Design review of the part built by this model. Coordinates are the model's own, in mm. A direction names the side the tool comes from. Coordinates: 2 decimals unless noted, no trailing zeros. Write each loop counter-clockwise with the first axis right and the second up, starting at its lowest first coordinate (ties: lowest second). Pieces come first, ordered by that corner, then holes. Notation, with made-up numbers: (-12.5, 85.25) -> (12.5, 85.25) arc R19 ccw to (12.5, 114.25) -> close; hole circle Ø11 at (72, 85.25). An arc over 180 degrees is marked (long way). One line per question, with ' | ' between items. Start each with the question number.
Q1. Draft analysis for pull direction X (two halves, no side actions). For faces 1 (the flat face through (4.762, 10, 2)), 2 (the flat face through (-9.525, -2, 2)), 3 (the flat face through (-4.762, 10, 2)), 4 (the flat face through (9.525, -2, 2)), state which applies: pulls with the +X half, pulls with the -X half, needs draft (parallel to the pull), parting line crosses it, or undercut.
Q2. Add section A-A on x = 0. State the section outline as (y, z) points (1 decimal).
Q3. For P1, Ø1, axis at y = -3, z = 1.5, coming from the +X side; P2, Ø1, axis at x = 8.5, z = 1, coming from the +Y side; P3, Ø1.6, axis at x = -8.5, z = 1.5, coming from the -Y side; P4, Ø10, axis at x = -8.5, y = 2.5, coming from the -Z side, all flat-tipped, find the tip position at first contact; note any pin that passes through.
Q4. Add section C-C on z = 2. Give the number of separate pieces and of enclosed holes in the cut face, and give its area (3 significant figures).
Q5. For faces 5 (the flat face through (-7, 7.938, 2)), 6 (the flat face through (7, 7.938, 2)), 7 (the flat face through (-6.35, -2, 2)), 8 (the flat face through (0, -3, 3.175)), list the 3-axis set-ups (+Z, -Z, +X, -X, +Y, -Y) from which the entire face can be reached by the end or side of a thin tool; tool diameter is ignored.
Q6. Add section D-D on y = 8.25. State the section outline as (x, z) points (1 decimal), and give its area (3 significant figures).
Q7. Wall thickness on probe 1 along X at (y, z) = (-13.5, 2.25); probe 2 along Y at (x, z) = (7, 2); probe 3 along X at (y, z) = (8, 3): over which ranges is each line inside the solid? List them lowest first.
Q8. Add section B-B on y = 0.5. State the section outline as (x, z) points (3 decimals).
from build123d import *

# Parameters (mm, degrees)
SKETCH1_W           = 9.525
SKETCH1_H           = 3.175
SKETCH1_R           = 2.38125
BOSS_EXTRUDE1_DEPTH = 3.175
CAVITY1_START       = -9.525
CAVITY1_OUTLINE_W   = 6.35
CAVITY1_OUTLINE_H   = 3.175
CAVITY1_DEPTH       = 3.175
CAVITY1_START_2     = 6.35
CAVITY1_2_OUTLINE_W = 6.35
CAVITY1_2_OUTLINE_H = 3.175
CAVITY1_2_DEPTH     = 3.175


# Read off the part's stored shape, not the designer's step: Cavity1
with BuildPart() as part:
    # Sketch1 → Boss-Extrude1 (new body)
    # profile 1 of 10: a face of its own
    with BuildSketch(Plane.XY):
        with BuildLine():
            ThreePointArc((-9.525, 7.9375), (-11.876811414, 4.274474566), (-12.7, 0))
            Line((-12.7, 0), (-9.525, 0))
            Line((-9.525, 0), (-9.525, 7.9375))
        make_face()
    # profile 2 of 10: a face of its own
    with BuildSketch(Plane.XY):
        with BuildLine():
            Line((-9.525, 0), (-12.7, 0))
            ThreePointArc((-12.7, 0), (-11.876811414, -4.274474566), (-9.525, -7.9375))
            Line((-9.525, -7.9375), (-9.525, 0))
        make_face()
    # profile 3 of 10: a face of its own
    with BuildSketch(Plane.XY):
        Polygon((-9.525, 7.9375), (-9.525, 0), (0, 0), (9.525, 0), (9.525, 7.9375), (4.7625, 7.9375), (-4.7625, 7.9375), align=None)
    # profile 4 of 10: a face of its own
    with BuildSketch(Plane.XY):
        Polygon((0, 0), (-9.525, 0), (-9.525, -7.9375), (0, -7.9375), (9.525, -7.9375), (9.525, 0), align=None)
    # profile 5 of 10: a face of its own
    with BuildSketch(Plane.XY):
        with BuildLine():
            Line((0, -7.9375), (-9.525, -7.9375))
            add(Edge.make_bspline(
                [(-9.525, -7.9375), (-8.354743729, -9.166269084), (-6.479229503, -10.75772626), (-5.396989703, -14.77189499), (-3.721125314, -16.086113374), (-2.300921541, -16.869792119)],
                knots=[0, 0, 0, 0, 0.40377748, 0.653864755, 1, 1, 1, 1], degree=3))
            ThreePointArc((-2.300921541, -16.869792119), (-4.611943257, -11.511982474), (0, -7.9375))
        make_face()
    # profile 6 of 10: a face of its own
    with BuildSketch(Plane.XY):
        with Locations((0, 9.525)):
            Rectangle(SKETCH1_W, SKETCH1_H)
    # profile 7 of 10: a face of its own
    with BuildSketch(Plane.XY):
        with BuildLine():
            Line((9.525, -7.9375), (0, -7.9375))
            ThreePointArc((0, -7.9375), (3.367596045, -9.332403955), (4.7625, -12.7))
            ThreePointArc((4.7625, -12.7), (4.1011916, -15.121081103), (2.300921541, -16.869792119))
            add(Edge.make_bspline(
                [(9.525, -7.9375), (8.354743729, -9.166269084), (6.479229503, -10.75772626), (5.396989703, -14.77189499), (3.721125314, -16.086113374), (2.300921541, -16.869792119)],
                knots=[0, 0, 0, 0, 0.40377748, 0.653864755, 1, 1, 1, 1], degree=3))
        make_face()
    # profile 8 of 10: a face of its own
    with BuildSketch(Plane.XY):
        with BuildLine():
            ThreePointArc((4.7625, -12.7), (3.367596045, -9.332403955), (0, -7.9375))
            ThreePointArc((0, -7.9375), (-4.611943257, -11.511982474), (-2.300921541, -16.869792119))
            ThreePointArc((-2.300921541, -16.869792119), (0, -17.4625), (2.300921541, -16.869792119))
            ThreePointArc((2.300921541, -16.869792119), (4.1011916, -15.121081103), (4.7625, -12.7))
        make_face()
        with Locations((0, -12.7)):
            Circle(SKETCH1_R, mode=Mode.SUBTRACT)
    # profile 9 of 10: a face of its own
    with BuildSketch(Plane.XY):
        with BuildLine():
            Line((9.525, 7.9375), (9.525, 0))
            Line((9.525, 0), (12.7, 0))
            ThreePointArc((12.7, 0), (11.876811414, 4.274474566), (9.525, 7.9375))
        make_face()
    # profile 10 of 10: a face of its own
    with BuildSketch(Plane.XY):
        with BuildLine():
            Line((12.7, 0), (9.525, 0))
            Line((9.525, 0), (9.525, -7.9375))
            ThreePointArc((9.525, -7.9375), (11.876811414, -4.274474566), (12.7, 0))
        make_face()
    extrude(amount=BOSS_EXTRUDE1_DEPTH)

    # Cavity1 outline → Cavity1 (cut)
    with BuildSketch(Plane.YZ.offset(CAVITY1_START)):
        with Locations((-1.5875, 1.5875)):
            Rectangle(CAVITY1_OUTLINE_W, CAVITY1_OUTLINE_H)
    extrude(amount=CAVITY1_DEPTH, mode=Mode.SUBTRACT)

    # Cavity1 2 outline → Cavity1 2 (cut)
    with BuildSketch(Plane.YZ.offset(CAVITY1_START_2)):
        with Locations((-1.5875, 1.5875)):
            Rectangle(CAVITY1_2_OUTLINE_W, CAVITY1_2_OUTLINE_H)
    extrude(amount=CAVITY1_2_DEPTH, mode=Mode.SUBTRACT)


solid = part.part
Output values:
1) face 1: pulls with the +X half | face 2: undercut | face 3: pulls with the -X half | face 4: undercut
2) outline: (-17.5, 0) -> (-15.1, 0) -> (-15.1, 3.2) -> (-17.5, 3.2) -> close; (-10.3, 0) -> (11.1, 0) -> (11.1, 3.2) -> (-10.3, 3.2) -> close
3) P1: stops at x = 12.43 | P2: stops at y = 7.94 | P3: stops at y = -9.82 | P4: stops at z = 0
4) separate pieces: 1 | enclosed holes: 3 | area: 456 mm2
5) face 5: +Z, -Z, -X, +Y | face 6: +Z, -Z, +X, +Y | face 7: +Z, -Z | face 8: +Z, +X, -X, +Y, -Y
6) outline: (-4.8, 0) -> (4.8, 0) -> (4.8, 3.2) -> (-4.8, 3.2) -> close | area: 30.2 mm2
7) probe 1: x = -5.65 to -2.24, 2.24 to 5.65 | probe 2: y = -10.69 to -4.76, 1.59 to 7.94 | probe 3: x = -4.76 to 4.76
8) outline: (-12.689, 0) -> (-9.525, 0) -> (-9.525, 3.175) -> (-12.689, 3.175) -> close; (-6.35, 0) -> (6.35, 0) -> (6.35, 3.175) -> (-6.35, 3.175) -> close; (9.525, 0) -> (12.689, 0) -> (12.689, 3.175) -> (9.525, 3.175) -> close
